from build123d import *

# Parameters (mm, degrees)
BOSS_EXTRUDE6_DEPTH = 25
SKETCH3_R           = 5
CUT_EXTRUDE1_DEPTH  = 96.096384068
SKETCH4_R           = 2.5
CUT_EXTRUDE2_DEPTH  = 96.096384068


with BuildPart() as part:
    # Sketch2 → Boss-Extrude6 (new body)
    with BuildSketch(Plane(origin=(0, 0, 0), x_dir=(0, 0, -1), z_dir=(1, 0, 0))):
        with BuildLine():
            Line((-32.496153619, -2.925741651), (-38, -2.925741651))
            ThreePointArc((-38, -2.925741651), (-67.69848481, -15.227256841), (-80, -44.925741651))
            Line((-80, -44.925741651), (-68, -44.925741651))
            ThreePointArc((-68, -44.925741651), (-59.213203436, -23.712538215), (-38, -14.925741651))
            Line((-38, -14.925741651), (-22.688150378, -14.925741651))
            Line((-22.688150378, -14.925741651), (26.657177064, -14.925741651))
            Line((26.657177064, -14.925741651), (26.657177064, 9.074258349))
            Line((26.657177064, 9.074258349), (-3.342822936, 9.074258349))
            ThreePointArc((-3.342822936, 9.074258349), (-16.948948047, 0.716384993), (-32.496153619, -2.925741651))
        make_face()
    extrude(amount=BOSS_EXTRUDE6_DEPTH)

    # Sketch3 → Cut-Extrude1 (cut, through all)
    with BuildSketch(Plane(origin=(25, 0, 0), x_dir=(0, 0, -1), z_dir=(1, 0, 0))):
        with Locations((8.657177064, -2.925741651)):
            Circle(SKETCH3_R)
    extrude(amount=-CUT_EXTRUDE1_DEPTH, mode=Mode.SUBTRACT)

    # Sketch4 → Cut-Extrude2 (cut, through all)
    with BuildSketch(Plane(origin=(25, 0, 0), x_dir=(0, 0, -1), z_dir=(1, 0, 0))):
        with Locations((-73.342822936, -37.425741651)):
            Circle(SKETCH4_R)
    extrude(amount=-CUT_EXTRUDE2_DEPTH, mode=Mode.SUBTRACT)


solid = part.part
Geometry check sheet. Reference: the model listing, model coordinates, mm. A direction names the side the tool comes from. Round coordinates to 2 decimals unless told otherwise and drop trailing zeros. Write each loop counter-clockwise with the first axis right and the second up, starting at its lowest first coordinate (ties: lowest second). Pieces come first, ordered by that corner, then holes. Notation, with made-up numbers: (70, 55.5) -> (115, 55.5) arc R26 cw to (115, 82.5) -> close; hole circle Ø5 at (-15.75, 32). An arc over 180 degrees is marked (long way). One line per item, written item: value. Start each with the question number.
(1) Go/stop test with flat-tipped pins: pin 1 Ø10 at (y, z) = (-20.5, 41.5) entering from -X; pin 2 Ø6 at (x, z) = (16.5, 21) entering from +Y; pin 3 Ø1.5 at (x, y) = (22, -32.5) entering from -Z; pin 4 Ø2 at (x, y) = (14.5, -24) entering from +Z. Record where each tip stops, or that it passes through.
(2) Access from +Z, -Z, +X, -X, +Y, -Y to the whole of each face (thin tool, end or side, straight path). Record for faces 1 (the cylindrical face through (12.675, -35.318, 71.999)), 2 (the flat face through (12, -14.926, 6)), 3 (the flat face through (12, -2.926, 35)).
(3) Cross-section at A-A, the plane y = -6. Record the cut outline in (x, z).
(4) Draft check along Z on faces 4 (the cylindrical face through (12.675, -4.841, -13.276)), 5 (the cylindrical face through (12.32, -14.9, 67.37)), 6 (the flat face through (12, 9.074, -12)). Enter one of: +Z half, -Z half, draft (parallel to the pull), parting line (faces both ways), or undercut.
(5) Cross-section at D-D, the plane z = 12. Record the cut outline in (x, y), and give its area (3 significant figures).
(6) Cross-section at B-B, the plane x = 2.75. Record the cut outline in (y, z).
(7) Scan lines: line 1 (Y direction, x = 14.5, z = 33.5); line 2 (Y direction, x = 23, z = -12); line 3 (Y direction, x = 1.5, z = 72). Record each from-to range of solid material in increasing order. Write a range as [from, to].
(8) Cross-section at C-C, the plane y = -0.5. Record the cut outline in (x, z), and give its area (3 significant figures).
Answer:
1. pin 1: through
1. pin 2: y = 0.3
1. pin 3: z = 64.95
1. pin 4: z = 74.97
2. face 1: +X, -X
2. face 2: -Z, +X, -X, -Y
2. face 3: +Z, +X, -X, +Y
3. outline: (0, -26.66) -> (25, -26.66) -> (25, -12.6) -> (0, -12.6) -> close; (0, -4.71) -> (25, -4.71) -> (25, 53.77) -> (0, 53.77) -> close
4. face 4: undercut
4. face 5: +Z half
4. face 6: draft
5. outline: (0, -14.93) -> (25, -14.93) -> (25, 3.08) -> (0, 3.08) -> close
5. area: 450 mm²
6. outline: (-44.93, 68) arc R30 cw to (-14.93, 38) -> (-14.93, -26.66) -> (9.07, -26.66) -> (9.07, 3.34) arc R50 cw to (-2.93, 32.5) -> (-2.93, 38) arc R42 ccw to (-44.93, 80) -> close; hole circle Ø5 at (-37.43, 73.34); hole circle Ø10 at (-2.93, -8.66)
7. line 1: [-14.93, -2.93]
7. line 2: [-14.93, -6.64], [0.79, 9.07]
7. line 3: [-44.93, -39.53], [-35.32, -20.27]
8. outline: (0, -26.66) -> (25, -26.66) -> (25, -13.03) -> (0, -13.03) -> close; (0, -4.29) -> (25, -4.29) -> (25, 20.22) -> (0, 20.22) -> close
8. area: 953 mm²
